For this review, take the finished solid that the model builds, in its own axes (mm). Face numbers are marked on the shaded views. A direction names the side the tool comes from. Give positions to 0.01 mm unless a question says otherwise; leave off trailing zeros. Order: outer loops, then holes, each group sorted by start corner. A loop starts at its lowest first (then second) coordinate and runs counter-clockwise, first axis right, second up. Notation, with made-up numbers: (-15, 70.25) -> (-8, 70.25) arc R24 cw to (-8, 97.25) -> close; hole circle Ø7 at (-7.75, 75). An arc over 180 degrees is marked (long way). Return JSON: item names as keys, results as strings. Group by question number.
1) To check wall thickness, follow line 1 along X through (y, z) = (0.85, 0); line 2 along Z through (x, y) = (0, 3.25); line 3 along X through (y, z) = (6.55, 0). State the ranges of each line that lie inside material, in increasing order.
2) Add section B-B (z = 0). State how many separate pieces and enclosed holes the cut face has, then the cut area to 3 significant figures.
3) Add section A-A (y = 2.25). Give the boundary of the cut face in (x, z), then the cut area to 3 significant figures.
4) For the marked faces 1, 2 and 3, list the 3-axis set-ups (+Z, -Z, +X, -X, +Y, -Y) from which the entire face can be reached by the end or side of a thin tool; tool diameter is ignored.
5) Insertion check: P1, Ø5, axis at x = -41.5, y = 3, coming from the +Z side; P2, Ø7, axis at x = 0, z = 0, coming from the +Y side; P3, Ø3.5, axis at y = 9, z = 1, coming from the +X side; P4, Ø4, axis at x = -36.5, y = 8.5, coming from the +Z side. Each pin has a flat end and moves straight along its axis. Give the tip position at first contact, or say it passes through.
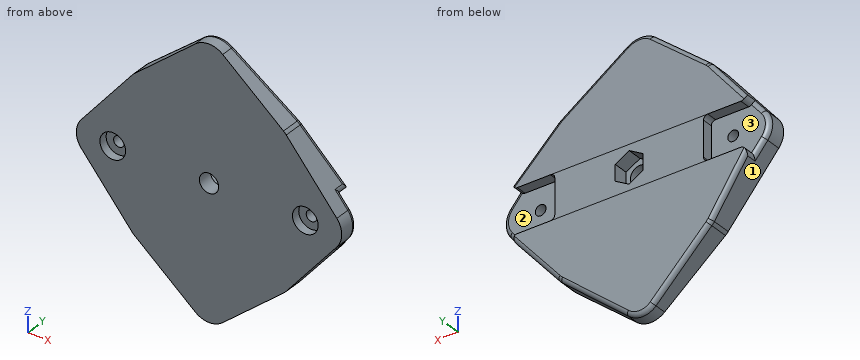
from build123d import *

# Parameters (mm, degrees)
ESQUISSE1_R                  = 4.5
ESQUISSE1_R_2                = 2.4999999999999947
ESQUISSE1_R_3                = 2.500000000000002
BOSS_EXTRU_1_DEPTH           = 9
ESQUISSE2_OUTSIDE_W          = 172.788
ESQUISSE2_OUTSIDE_H          = 199.11
ENL_V_MAT_EXTRU_1_DEPTH      = 103.10046824457444
CONG_1_R                     = 10
ESQUISSE3_R                  = 4.5
BOSS_EXTRU_2_DEPTH           = 5
ENL_V_MAT_EXTRU_2_DEPTH      = 7
ESQUISSE5_R                  = 6.000000000000003
ENL_V_MAT_EXTRU_3_DEPTH      = 4
ENL_V_MAT_EXTRU_5_DEPTH      = 116.79687329576521
ENL_V_MAT_EXTRU_5_DEPTH_BACK = 116.79687329576521
CONG_2_R                     = 2


with BuildPart() as part:
    # Esquisse1 → Boss.-Extru.1 (new body)
    with BuildSketch(Plane(origin=(0, 0, 0), x_dir=(1, 0, 0), z_dir=(0, 1, 0))):
        Polygon((-65.03288181544035, -1.1e-16), (1.14e-14, -78.19354128404926), (65.03288181544036, -2.2e-16), (-1.33e-15, 78.19354128404929), align=None)
        with Locations(Location((0, 0, 0), (0, 0, 270))):
            Circle(ESQUISSE1_R, mode=Mode.SUBTRACT)
        with Locations(Location((-45, 0, 0), (0, 0, 270))):
            Circle(ESQUISSE1_R_2, mode=Mode.SUBTRACT)
        with Locations(Location((45, 0, 0), (0, 0, 270))):
            Circle(ESQUISSE1_R_3, mode=Mode.SUBTRACT)
    extrude(amount=BOSS_EXTRU_1_DEPTH)

    # Esquisse2 outside → Enlèv. mat.-Extru.1 (cut, through all)
    with BuildSketch(Plane(origin=(0, 9, 0), x_dir=(1, 0, 0), z_dir=(0, 1, 0))):
        Rectangle(ESQUISSE2_OUTSIDE_W, ESQUISSE2_OUTSIDE_H)
        Polygon((3.05e-15, 65.03288181544038), (-78.1935412840493, 1.183e-14), (-1.388e-14, -65.03288181544033), (78.1935412840493, 1.69e-14), align=None, mode=Mode.SUBTRACT)
    extrude(amount=-ENL_V_MAT_EXTRU_1_DEPTH, mode=Mode.SUBTRACT)

    # Congé1
    cong_1_edges = [part.edges().sort_by_distance(p)[0] for p in [
        (35.50428209412193, 4.5, -35.50428209412183),
        (35.504282094121805, 4.5, 35.50428209412193),
        (-35.50428209412127, 4.5, 35.50428209412245),
        (-35.504282094121926, 4.5, -35.504282094121834),
        (3.05e-15, 4.5, -65.03288181544038),
        (-1.388e-14, 4.5, 65.03288181544033),
        (65.03288181544036, 4.5, 2.2e-16),
        (-65.03288181544035, 4.5, 1.1e-16),
    ]]
    fillet(cong_1_edges, radius=CONG_1_R)

    # Esquisse3 → Boss.-Extru.2 (add)
    with BuildSketch(Plane(origin=(0, 9, 0), x_dir=(1, 0, 0), z_dir=(0, 1, 0))):
        with BuildLine():
            Line((-56.50804680142313, 10.250000000000002), (-34.74999999999999, 10.25))
            Line((-34.74999999999999, 10.25), (-34.74999999999999, -10.25))
            Line((-34.74999999999999, -10.25), (-56.50804680142313, -10.25))
            Line((-56.50804680142313, -10.25), (-36.091843996032054, -34.79781569510337))
            ThreePointArc((-36.091843996032054, -34.79781569510337), (-35.47449348716292, -35.47449348716301), (-34.79781569510328, -36.091843996032146))
            Line((-34.79781569510328, -36.091843996032146), (-6.394390019805823, -59.71472377308688))
            ThreePointArc((-6.394390019805823, -59.71472377308688), (-2.16e-15, -62.026305452352254), (6.3943900198058135, -59.71472377308687))
            Line((6.3943900198058135, -59.71472377308687), (34.797815695103374, -36.09184399603205))
            ThreePointArc((34.797815695103374, -36.09184399603205), (35.47449348716302, -35.47449348716292), (36.09184399603216, -34.79781569510327))
            Line((36.09184399603216, -34.79781569510327), (56.50804680142313, -10.25))
            Line((56.50804680142313, -10.25), (34.74999999999999, -10.25))
            Line((34.74999999999999, -10.25), (34.74999999999999, 10.25))
            Line((34.74999999999999, 10.25), (56.50804680142313, 10.250000000000002))
            Line((56.50804680142313, 10.250000000000002), (36.09184399603206, 34.797815695103395))
            ThreePointArc((36.09184399603206, 34.797815695103395), (35.47449348716294, 35.47449348716303), (34.7978156951033, 36.09184399603216))
            Line((34.7978156951033, 36.09184399603216), (6.394390019805837, 59.71472377308691))
            ThreePointArc((6.394390019805837, 59.71472377308691), (5.05e-15, 62.02630545235231), (-6.394390019805832, 59.71472377308692))
            Line((-6.394390019805832, 59.71472377308692), (-34.797815695103225, 36.09184399603222))
            ThreePointArc((-34.797815695103225, 36.09184399603222), (-35.47449348716287, 35.47449348716309), (-36.091843996032004, 34.79781569510345))
            Line((-36.091843996032004, 34.79781569510345), (-56.50804680142313, 10.250000000000002))
        make_face()
        with Locations(Location((0, 0, 0), (0, 0, 270))):
            Circle(ESQUISSE3_R, mode=Mode.SUBTRACT)
    extrude(amount=BOSS_EXTRU_2_DEPTH)

    # Esquisse4 → Enlèv. mat.-Extru.2 (cut)
    with BuildSketch(Plane(origin=(0, 13.999999999999998, 0), x_dir=(1, 0, 0), z_dir=(0, 1, 0))):
        Polygon((6.500000000000003, 3.7527767497325644), (3.51e-15, 7.5055534994651305), (-6.499999999999996, 3.752776749732566), (-6.499999999999996, -3.752776749732568), (7.1e-15, -7.505553499465138), (6.499999999999999, -3.752776749732574), align=None)
    extrude(amount=-ENL_V_MAT_EXTRU_2_DEPTH, mode=Mode.SUBTRACT)

    # Esquisse5 → Enlèv. mat.-Extru.3 (cut)
    with BuildSketch(Plane.XZ):
        with Locations(Location((-45, 0, 0), (0, 0, 270))):
            Circle(ESQUISSE5_R)
        with Locations(Location((45, 0, 0), (0, 0, 270))):
            Circle(ESQUISSE5_R)
    extrude(amount=-ENL_V_MAT_EXTRU_3_DEPTH, mode=Mode.SUBTRACT)

    # Esquisse6 → Enlèv. mat.-Extru.5 (cut, two sides: drawn at the far end of the back side and taken through both)
    with BuildSketch(Plane(origin=(34.74999999999999, 0, 0), x_dir=(0, 0, -1), z_dir=(1, 0, 0)).offset(-ENL_V_MAT_EXTRU_5_DEPTH_BACK)):
        Polygon((-62.02630545235226, 6.999999999999998), (-10.25, 13.999999999999998), (10.25, 13.999999999999998), (62.02630545235227, 7.000000000000001), (62.026305452352254, 36.4147856499244), (-62.026305452352254, 36.4147856499244), align=None)
    extrude(amount=ENL_V_MAT_EXTRU_5_DEPTH + ENL_V_MAT_EXTRU_5_DEPTH_BACK, mode=Mode.SUBTRACT)

    # Congé2
    cong_2_edges = [part.edges().sort_by_distance(p)[0] for p in [
        (58.11138528725502, 9, 8.322195009902927),
        (-58.11138528725501, 9, -8.322195009902927),
        (56.50804680142313, 11.5, 10.25),
        (34.74999999999999, 11.5, 10.25),
        (34.74999999999999, 11.5, -10.25),
        (56.50804680142313, 11.5, -10.250000000000002),
        (-56.50804680142313, 11.5, -10.250000000000002),
        (-34.74999999999999, 11.5, -10.25),
        (-34.74999999999999, 11.5, 10.25),
        (-56.50804680142313, 11.5, 10.25),
        (-46.299945398727594, 12.340604757673788, -22.523907847551726),
        (46.2999453987276, 12.340604757673791, -22.523907847551705),
        (20.596102857454603, 8.909389828239629, -47.90328388455951),
        (3.4028602353834634, 7.0806828820281655, -61.429525231685666),
        (35.47476156274495, 10.589760967545045, -35.47422540141744),
        (-46.299945398727345, 12.340604757673752, 22.523907847551982),
        (46.29994539872759, 12.340604757673788, 22.523907847551698),
        (3.4028602353834314, 7.080682882028164, 61.429525231685645),
        (20.596102857454596, 8.909389828239629, 47.903283884559464),
        (35.4747615627448, 10.589760967545022, 35.47422540141758),
        (-20.596102857454614, 8.909389828239625, -47.903283884559514),
        (-35.47476156274494, 10.589760967545041, -35.47422540141746),
        (-35.47476156274429, 10.589760967544956, 35.474225401418074),
        (-20.59610285745456, 8.909389828239624, 47.90328388455953),
        (58.11138528725502, 9, -8.322195009902925),
        (-58.111385287255004, 9, 8.322195009902918),
        (-62.02630545235229, 9, 8.38e-15),
        (62.02630545235229, 9, -4.51e-15),
    ]]
    fillet(cong_2_edges, radius=CONG_2_R)


solid = part.part
Evaluation:
{
 "1": {"line 1": "-62.03 to -51, -39 to -4.5, 4.5 to 39, 51 to 62.03", "line 2": "-62.03 to -4.5, 4.5 to 62.03", "line 3": "-62.03 to -47.5, -42.5 to -4.5, 4.5 to 42.5, 47.5 to 62.03"},
 "2": {"separate pieces": "4", "enclosed holes": "0", "area": "1,160 mm^2"},
 "3": {"outline": "(-59.71, -6.39) -> (-36.09, -34.8) arc R10 ccw to (-34.8, -36.09) -> (-6.39, -59.71) arc R10 ccw to (6.39, -59.71) -> (34.8, -36.09) arc R10 ccw to (36.09, -34.8) -> (59.71, -6.39) arc R10 ccw to (59.71, 6.39) -> (36.09, 34.8) arc R10 ccw to (34.8, 36.09) -> (6.39, 59.71) arc R10 ccw to (-6.39, 59.71) -> (-34.8, 36.09) arc R10 ccw to (-36.09, 34.8) -> (-59.71, 6.39) arc R10 ccw to start; hole circle Ø12 at (-45, 0); hole circle Ø9 at (0, 0); hole circle Ø12 at (45, 0)", "area": "8,890 mm^2"},
 "4": {"face 1": "-Z, -X, +Y, -Y", "face 2": "+X, +Y", "face 3": "-X, +Y"},
 "5": {"P1": "z = 31.3", "P2": "through", "P3": "x = 61.99", "P4": "z = 36.34"}
}
